Part model, mm, in its own coordinate system. A direction names the side the tool comes from. Give positions to 0.01 mm unless a question says otherwise; leave off trailing zeros. Write each loop counter-clockwise with the first axis right and the second up, starting at its lowest first coordinate (ties: lowest second). Pieces come first, ordered by that corner, then holes. Notation, with made-up numbers: M 4,-5 L 59,-5 A23 cw 59,9 Z; hole C 66,51 d1. An arc over 180 degrees is marked long. Answer as CSV lines item,"result". Start each with the question number.
1) Slice it at A-A, the plane z = 268.5. Give the cut face in (x, y).
2) Slice it at B-B, the plane z = 480. Give the cut face in (x, y), plus the area to 3 significant figures.
3) Slice it at D-D, the plane x = 114. Give the cut face in (y, z), plus the area to 3 significant figures.
4) Mould opens along Y. For faces 1 (the flat face through (-49, -153.29, 350.15)), 2 (the flat face through (-191, 196.71, 551)), 3 (the flat face through (-176, -128, 0)) say: pulls with the +Y half, pulls with the -Y half, needs draft (parallel to the pull), parting line crosses it, or undercut.
5) Pin check, flat tips, straight feed: pin 1 Ø12 at (x, y) = (39, 140.5) entering from -Z; pin 2 Ø2 at (x, y) = (-57.5, 46) entering from +Z. Stop position of each tip, or through.
6) Tool access for faces 4 (the flat face through (-207.205, -128.64, 700.933)), 5 (the flat face through (-176, 196.71, 173)), 6 (the flat face through (149.638, -129, 173)): list every direction of +Z, -Z, +X, -X, +Y, -Y with a clear straight run to the whole face (end or side of a thin tool).
7) Wall check: line 1 along X through (y, z) = (-132, 259); line 2 along Y through (x, z) = (151, 133); line 3 along Z through (x, y) = (-151, -101). Give the ranges that are in metal, low to high. Write a range as from..to.
8) Slice it at C-C, the plane y = 216.5. Give the cut face in (x, z).
```python
from build123d import *

# Parameters (mm, degrees)
F0_W      = 400
F0_H      = 400
F1_DEPTH  = 400
F2_W      = 300
F2_H      = 350
F3_DEPTH  = 400
F4_W      = 300
F4_H      = 350
F5_DEPTH  = 400
F6_W      = 50
F6_H      = 400
F7_DEPTH  = 300
F8_W      = 300
F8_H      = 300
F9_DEPTH  = 50
F10_DEPTH = 300
F11_DEPTH = 300
F15_W     = 50
F15_H     = 300
F16_DEPTH = 50
F17_DEPTH = 25
F18_W     = 50
F18_H     = 300
F19_DEPTH = 50
F20_DEPTH = 5.2552117633


with BuildPart() as f1:
    # F0 (on Top) → F1 (new body)
    with BuildSketch(Plane.XY):
        with Locations((-0.3617890179, 46.7100545251)):
            Rectangle(F0_W, F0_H)
    extrude(amount=F1_DEPTH)

    # F2 (on face) → F3 (cut)
    with BuildSketch(Plane(origin=(-200.3617890179, 0, 0), x_dir=(0, -1, 0), z_dir=(-1, 0, 0))):
        with Locations((-46.7100545251, 175)):
            Rectangle(F2_W, F2_H)
    extrude(amount=-F3_DEPTH, mode=Mode.SUBTRACT)

    # F4 (on face) → F5 (cut)
    with BuildSketch(Plane.XZ.offset(153.2899454749)):
        with Locations((-0.3617890179, 175)):
            Rectangle(F4_W, F4_H)
    extrude(amount=-F5_DEPTH, mode=Mode.SUBTRACT)

    # F6 (on face) → F7 (join)
    with BuildSketch(Plane.XY.offset(400)):
        with Locations((-175.3617890179, 46.7100545251)):
            Rectangle(F6_W, F6_H)
    extrude(amount=F7_DEPTH)

    # F8 (on face) → F9 (cut)
    with BuildSketch(Plane.YZ.offset(-150.3617890179)):
        with Locations((46.7100545251, 550)):
            Rectangle(F8_W, F8_H)
    extrude(amount=-F9_DEPTH, mode=Mode.SUBTRACT)

    # F10 (cut): a face of the model
    f10_faces = [f1.faces().sort_by_distance(p)[0] for p in [
        (-175.3617890179, -128.2899454749, 700),
    ]]
    extrude(f10_faces, amount=-F10_DEPTH, mode=Mode.SUBTRACT)

    # F11 (cut): a face of the model
    f11_faces = [f1.faces().sort_by_distance(p)[0] for p in [
        (-175.3617890179, 221.7100545251, 700),
    ]]
    extrude(f11_faces, amount=-F11_DEPTH, mode=Mode.SUBTRACT)

    # F15 (on face) → F16 (join)
    with BuildSketch(Plane(origin=(-156.5902579487, 0, -16.4582993118), x_dir=(0, 1, 0), z_dir=(0.9945218954, 0, 0.1045284633))):
        with Locations((-128.2899454749, 568.7522680509)):
            Rectangle(F15_W, F15_H)
    extrude(amount=F16_DEPTH)

    # F17 (add): a face of the model
    f17_faces = [f1.faces().sort_by_distance(p)[0] for p in [
        (-175.4987416337, -128.2899454749, 402.6132115817),
    ]]
    extrude(f17_faces, amount=F17_DEPTH)



with BuildPart() as f19:
    # F18 (on face) → F19 (new body)
    with BuildSketch(Plane(origin=(-156.5902579487, 0, -16.4582993118), x_dir=(0, 1, 0), z_dir=(0.9945218954, 0, 0.1045284633))):
        with Locations((221.7100545251, 568.7522680509)):
            Rectangle(F18_W, F18_H)
    extrude(amount=F19_DEPTH)


with BuildPart() as f1_1:
    add(f1.part)
    # F20 (add, through all): a face of the model
    f20_faces = [f19.part.faces().sort_by_distance(p)[0] for p in [
        (-175.4987416337, 221.7100545251, 402.6132115817),
    ]]

    add(f19.part)  # F20 merges F19
    extrude(f20_faces, amount=F20_DEPTH)


solid = f1_1.part
```
Found:
1,outline,"M -200.36,-153.29 L -150.36,-153.29 L -150.36,-103.29 L -200.36,-103.29 Z; M -200.36,196.71 L -150.36,196.71 L -150.36,246.71 L -200.36,246.71 Z; M 149.64,-153.29 L 199.64,-153.29 L 199.64,-103.29 L 149.64,-103.29 Z; M 149.64,196.71 L 199.64,196.71 L 199.64,246.71 L 149.64,246.71 Z"
2,outline,"M -208.77,-153.29 L -158.49,-153.29 L -158.49,-103.29 L -208.77,-103.29 Z; M -208.77,196.71 L -158.49,196.71 L -158.49,246.71 L -208.77,246.71 Z"
2,area,"5,030 mm²"
3,outline,"M -153.29,350 L 246.71,350 L 246.71,400 L -153.29,400 Z"
3,area,"20,000 mm²"
4,face 1,"pulls with the -Y half"
4,face 2,"undercut"
4,face 3,"needs draft"
5,pin 1,"z = 350"
5,pin 2,"z = 400"
6,face 4,"+Z, -X, +Y, -Y"
6,face 5,"-Z, +X, -X"
6,face 6,"-Z, +Y, -Y"
7,line 1,"-200.36..-150.36, 149.64..199.64"
7,line 2,"-153.29..-103.29, 196.71..246.71"
7,line 3,"350..400"
8,outline,"M -231.72,698.36 L -200.36,400 L -200.36,0 L -150.36,0 L -150.36,350 L 149.64,350 L 149.64,0 L 199.64,0 L 199.64,400 L -150.09,400 L -181.99,703.58 Z"
